Job drawing, mm, ordinate dimensions from the low corner. One solid piece. A direction names the side the tool comes from. Round coordinates to 2 decimals unless told otherwise and drop trailing zeros. Loops run counter-clockwise (first coordinate to the right, second up) from the corner with the lowest first, then second, coordinate; pieces in that order, holes last. Notation, with made-up numbers: M -38,-39 L -5,-39 A30 cw -5,-17 Z; hole C 54,-39.5 d9. An arc over 180 degrees is marked long. Put each result on its own line as item: value. Start each with the question number.
1) Probe line 1 along X through (y, z) = (94, 267); line 2 along X through (y, z) = (93, 528.5); line 3 along Z through (x, y) = (109.5, 66.5) (1 decimal). List the from-to ranges inside material, lowest first.
2) Drop flat-ended pins along their axis: pin 1 Ø6 at (x, z) = (100.5, 156) entering from -Y; pin 2 Ø5 at (x, y) = (88, 35.5) entering from +Z; pin 3 Ø12 at (x, y) = (51, 121.5) entering from -Z. Give the stop position or say it passes through.
3) Slice it at A-A on z = 360.5. Give the cut face in (x, y).
4) Which spindle directions (+Z, -Z, +X, -X, +Y, -Y) get a long thin tool onto all of the face, cutting with end or side? Do the marked faces 1 and 2. Say none if no direction does.
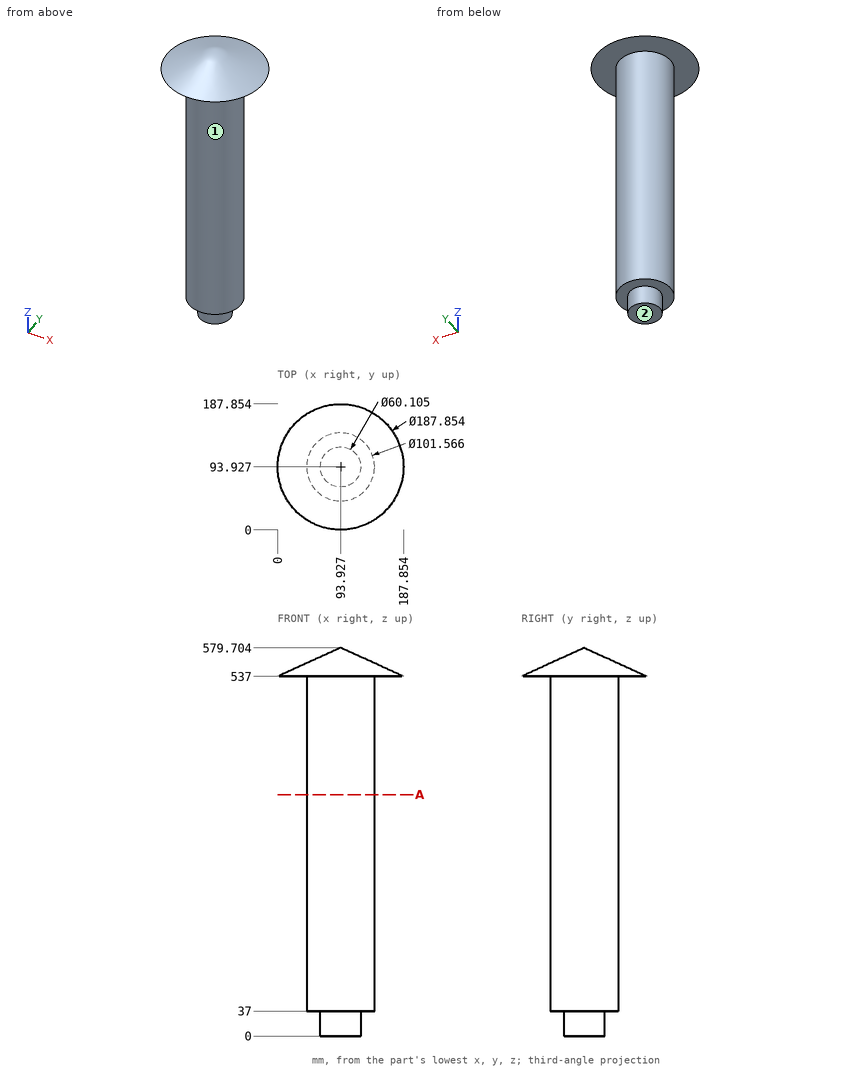
Recorded:
1. line 1: x = 43.14 to 144.71
1. line 2: x = 43.15 to 144.7
1. line 3: z = 37 to 565.4
2. pin 1: stops at y = 43.27
2. pin 2: stops at z = 554.14
2. pin 3: stops at z = 37
3. outline: C 93.93,93.93 d101.57
4. face 1: -Z
4. face 2: -Z, +X, -X, +Y, -Y
